from build123d import *
from OCP.BRepFilletAPI import BRepFilletAPI_MakeChamfer

# Parameters (mm, degrees)
SKETCH1_W           = 20
SKETCH1_H           = 22
BOSS_EXTRUDE1_DEPTH = 25
CIRPATTERN1_COUNT   = 5
CIRPATTERN1_ANGLE   = 130
CHAMFER1_SIZE       = 15
CHAMFER1_SIZE2      = 8.660254038
CHAMFER3_SIZE       = 10
CHAMFER3_SIZE2      = 5.773502692


with BuildPart() as part:
    # Sketch1 → Boss-Extrude1 (new body)
    with BuildSketch(Plane.XY):
        with BuildLine():
            Line((-150, 0), (0, 0))
            ThreePointArc((0, 0), (-75, -75), (-150, 0))
        make_face()
        with Locations((-55.5, -26)):
            Rectangle(SKETCH1_W, SKETCH1_H, mode=Mode.SUBTRACT)
        with Locations((-94.5, -26)):
            Rectangle(SKETCH1_W, SKETCH1_H, mode=Mode.SUBTRACT)
    extrude(amount=BOSS_EXTRUDE1_DEPTH)

    # Sketch4 → Ø4.0mm Dowel Hole2 (revolve, cut)
    with BuildSketch(Plane(origin=(-7.026915972, -31.696369631, 12.5), x_dir=(0.4226182617407001, 0.9063077870366498, 0), z_dir=(0, 0, 1))):
        Polygon((0, 0), (0, 17.201721238), (2, 16), (2, 0.025), (2.025, 0), align=None)
    f_4_0mm_dowel_hole2 = revolve(axis=Axis((-1.271861525, -34.379995593, 12.5), (-0.9063077870366496, 0.42261826174070005, 0)), mode=Mode.SUBTRACT)

    # CirPattern1: Ø4.0mm Dowel Hole2 ×5 about axis
    cirpattern1_axis = Axis((-75, 0, 0), (0, 0, -1))
    for i in range(1, CIRPATTERN1_COUNT):
        add(f_4_0mm_dowel_hole2.rotate(cirpattern1_axis, i * CIRPATTERN1_ANGLE / (CIRPATTERN1_COUNT - 1)), mode=Mode.SUBTRACT)

    # Chamfer1: one chamfer whose edges measure the first distance from different faces: ONE call of the kernel's chamfer builder (chamfer() names one face for all edges)
    chamfer1_edges_1 = [part.edges().sort_by_distance(p)[0] for p in [
        (-55.5, -15, 0),
    ]]
    chamfer1_side_1 = [part.faces().sort_by_distance(p)[0] for p in [
        (-55.5, -15, 12.5),
    ]]
    chamfer1_edges_2 = [part.edges().sort_by_distance(p)[0] for p in [
        (-94.5, -15, 0),
    ]]
    chamfer1_side_2 = [part.faces().sort_by_distance(p)[0] for p in [
        (-94.5, -15, 12.5),
    ]]
    chamfer1 = BRepFilletAPI_MakeChamfer(part.part.solid().wrapped)
    for e in chamfer1_edges_1:
        chamfer1.Add(CHAMFER1_SIZE, CHAMFER1_SIZE2, e.wrapped, chamfer1_side_1[0].wrapped)  # the first distance lies on this face
    for e in chamfer1_edges_2:
        chamfer1.Add(CHAMFER1_SIZE, CHAMFER1_SIZE2, e.wrapped, chamfer1_side_2[0].wrapped)  # the first distance lies on this face
    add(Compound.cast(chamfer1.Shape()), mode=Mode.REPLACE)

    # Chamfer3: one chamfer whose edges measure the first distance from different faces: ONE call of the kernel's chamfer builder (chamfer() names one face for all edges)
    chamfer3_edges_1 = [part.edges().sort_by_distance(p)[0] for p in [
        (-104.5, -26, 25),
    ]]
    chamfer3_side_1 = [part.faces().sort_by_distance(p)[0] for p in [
        (-104.5, -24.533265853, 11.707841645),
    ]]
    chamfer3_edges_2 = [part.edges().sort_by_distance(p)[0] for p in [
        (-84.5, -26, 25),
    ]]
    chamfer3_side_2 = [part.faces().sort_by_distance(p)[0] for p in [
        (-84.5, -24.533265853, 11.707841645),
    ]]
    chamfer3_edges_3 = [part.edges().sort_by_distance(p)[0] for p in [
        (-45.5, -26, 25),
    ]]
    chamfer3_side_3 = [part.faces().sort_by_distance(p)[0] for p in [
        (-45.5, -24.533265853, 11.707841645),
    ]]
    chamfer3_edges_4 = [part.edges().sort_by_distance(p)[0] for p in [
        (-65.5, -26, 25),
    ]]
    chamfer3_side_4 = [part.faces().sort_by_distance(p)[0] for p in [
        (-65.5, -24.533265853, 11.707841645),
    ]]
    chamfer3 = BRepFilletAPI_MakeChamfer(part.part.solid().wrapped)
    for e in chamfer3_edges_1:
        chamfer3.Add(CHAMFER3_SIZE, CHAMFER3_SIZE2, e.wrapped, chamfer3_side_1[0].wrapped)  # the first distance lies on this face
    for e in chamfer3_edges_2:
        chamfer3.Add(CHAMFER3_SIZE, CHAMFER3_SIZE2, e.wrapped, chamfer3_side_2[0].wrapped)  # the first distance lies on this face
    for e in chamfer3_edges_3:
        chamfer3.Add(CHAMFER3_SIZE, CHAMFER3_SIZE2, e.wrapped, chamfer3_side_3[0].wrapped)  # the first distance lies on this face
    for e in chamfer3_edges_4:
        chamfer3.Add(CHAMFER3_SIZE, CHAMFER3_SIZE2, e.wrapped, chamfer3_side_4[0].wrapped)  # the first distance lies on this face
    add(Compound.cast(chamfer3.Shape()), mode=Mode.REPLACE)


solid = part.part
Geometry check sheet. Reference: the model listing, model coordinates, mm. A direction names the side the tool comes from. Give positions to 0.01 mm unless a question says otherwise; leave off trailing zeros. Write each loop counter-clockwise with the first axis right and the second up, starting at its lowest first coordinate (ties: lowest second). Pieces come first, ordered by that corner, then holes. Notation, with made-up numbers: (40.25, -2) - (69.25, -2) arc R24 cw to (69.25, 33) - close; hole circle Ø5 at (-20.5, -19.75). An arc over 180 degrees is marked (long way). Put each result on its own line as item: value.
1. Sectioned sample at D-D, the plane y = -44.5. Enter the section's corners in (x, z).
Ans:
outline: (-135.37, 0) - (-14.63, 0) - (-14.63, 25) - (-135.37, 25) - close
2. Draft check along X on faces 1 (the cylindrical face through (-135.01, -30.09, 11.9)), 2 (the flat face through (-56, -37, 12)), 3 (the flat face through (-76, 0, 12)). Enter one of: +X half, -X half, draft (parallel to the pull), parting line (faces both ways), or undercut.
Ans:
face 1: undercut
face 2: undercut
face 3: draft
3. Sectioned sample at B-B, the plane x = -99. Enter the section's corners in (y, z).
Ans:
outline: (-71.06, 0) - (-37, 0) - (-37, 25) - (-71.06, 25) - close; (-15, 15) - (-6.34, 0) - (0, 0) - (0, 25) - (-15, 25) - close
4. Sectioned sample at C-C, the plane z = 17.5. Enter the section's corners in (x, y), plus the area to 3 significant figures.
Ans:
outline: (-150, 0) arc R75 ccw to (0, 0) - close; hole (-105.94, -37) - (-83.06, -37) - (-83.06, -15) - (-105.94, -15) - close; hole (-66.94, -37) - (-44.06, -37) - (-44.06, -15) - (-66.94, -15) - close
area: 7,830 mm²
5. Thickness scan on line 1 (Z direction, x = -75, y = -70.75); line 2 (X direction, y = -32, z = 23.25); line 3 (Y direction, x = -95, z = 22). Record the ranges inside material, lowest first.
Ans:
line 1: z = 0 to 10.5, 14.5 to 25
line 2: x = -142.83 to -109.26, -79.74 to -70.26, -40.74 to -7.17
line 3: y = -72.28 to -37, -15 to 0
6. Sectioned sample at A-A, the plane y = -17.5. Enter the section's corners in (x, z).
Ans:
outline: (-147.93, 0) - (-104.5, 0) - (-104.5, 15) - (-110.27, 25) - (-147.93, 25) - close; (-84.5, 0) - (-65.5, 0) - (-65.5, 15) - (-71.27, 25) - (-78.73, 25) - (-84.5, 15) - close; (-45.5, 0) - (-2.07, 0) - (-2.07, 25) - (-39.73, 25) - (-45.5, 15) - close
7. Go/stop test with flat-tipped pins: pin 1 (1.5 mm diameter, centred on x = -127.5, z = 13.5, fed in from -Y); pin 2 (5 mm diameter, centred on x = -52.5, z = 21, fed in from -Y); pin 3 (1.5 mm diameter, centred on y = -60.5, z = 12.5, fed in from -X). Record where each tip stops, or that it passes through.
Ans:
pin 1: stops at y = -54.29
pin 2: stops at y = -72.28
pin 3: stops at x = -120.33
8. Set-up check for faces 4 (the cylindrical face through (-76.998, -67.099, 12.412)), 5 (the flat face through (-55.64, -10.609, 7.395)), 6 (the conical face through (-22.288, -24.215, 12.396)), 7 (the flat face through (-74, -29, 25)), 8 (the flat face through (-81.573, -26.154, 20.07)): record each of +Z, -Z, +X, -X, +Y, -Y from which the full face is reachable in a straight line by a thin tool's end or side.
Ans:
face 4: -Y
face 5: -Z
face 6: none
face 7: +Z, +X, -X, +Y, -Y
face 8: +Z
